Work out the finished part from the listing and answer in its coordinate system (mm). Face numbers are marked on the shaded views. A direction names the side the tool comes from. Coordinates: 2 decimals unless noted, no trailing zeros. Loops run counter-clockwise (first coordinate to the right, second up) from the corner with the lowest first, then second, coordinate; pieces in that order, holes last. Notation, with made-up numbers: (2.5, 23.25) -> (7.5, 23.25) arc R27 cw to (7.5, 54.25) -> close; hole circle Ø5 at (-2, 18). An arc over 180 degrees is marked (long way). Use a Markdown table: item, result. Add a question column.
Autodesk Inventor part; units mm, degrees
ref_plane "Work Plane1" through (-60, 0, 0) normal (1, 0, 0) x (0, 1, 0)
ref_plane "XZ Plane" through (0, 0, 0) normal (0, 1, 0) x (-1, 0, 0)
ref_plane "XY Plane" through (0, 0, 0) normal (0, 0, 1) x (1, 0, 0)
sketch "Sketch1" plane through (0, 0, 0) normal (0, 0, 1) x (1, 0, 0)
  circle A0 centre (0, 0) radius 25
  line L0 (0, 25) -> (-60, 25)
  line L1 (0, -25) -> (-60, -25)
  arc A1 (-60, 25) -> (-60, -25) centre (-60, 0) ccw
  dimension "d0" = 50
  dimension "d1" = 60
  dimension "d2" = 60
  dimension "d3" = 25
extrude "Extrusion1" add sketch "Sketch1" along normal mid plane 93
sketch "Sketch2" plane through (0, 0, 0) normal (0, 0, 1) x (1, 0, 0)
  arc A0 (0, -25) -> (0, 25) centre (0, 0) ccw
  arc A1 (-12.2474, 25) -> (-11.5542, 22.1698) centre (-12.2474, 23.5) ccw construction
  arc A2 (-11.5542, -22.1698) -> (-12.2474, -25) centre (-12.2474, -23.5) ccw construction
  line L0 (0, -25) -> (-60, -25)
  line L1 (-60, 25) -> (0, 25)
  line L2 (-12.2474, 25) -> (0, 25)
  arc A3 (0, -25) -> (0, 25) centre (0, 0) ccw
  line L3 (-12.2474, -25) -> (0, -25)
  arc A4 (-11.5542, -22.1698) -> (0, -25) centre (0, 0) ccw construction
  arc A5 (-12.2474, -25) -> (-11.5542, -22.1698) centre (-12.2474, -23.5) ccw
  arc A6 (-11.5542, 22.1698) -> (-12.2474, 25) centre (-12.2474, 23.5) ccw
  arc A7 (-11.5542, 22.1698) -> (-11.5542, -22.1698) centre (0, 0) ccw
  arc A8 (0, 25) -> (-11.5542, 22.1698) centre (0, 0) ccw construction
  dimension "d7" = 3
  dimension "d8" = 3
extrude "Extrusion2" cut sketch "Sketch2" along normal mid plane 78
sketch "Sketch3" plane through (0, 0, 0) normal (0, 0, 1) x (1, 0, 0)
  circle A0 centre (0, 0) radius 10
  dimension "d11" = 20
extrude "Extrusion3" cut sketch "Sketch3" along normal mid plane 88
sketch "Sketch4" plane through (-60, 25, -46.5) normal (0, 1, 0) x (1, 0, 0)
  line L0 (35, -7.5) -> (35, -85.5)
  line L1 (0, -93) -> (60, -93)
  line L2 (30, -93) -> (30, 0)
  line L3 (60, 0) -> (0, 0)
  line L4 (30, -93) -> (-25, -71.5)
  line L5 (-25, 0) -> (-25, -93)
  line L6 (-25, -71.5) -> (-25, -93)
  line L7 (30, -93) -> (-25, -93)
  line L8 (30, 0) -> (-25, -21.5)
  line L9 (-25, 0) -> (30, 0)
  line L10 (-25, -21.5) -> (-25, 0)
  point P0 (60, -46.5)
  dimension "d14" = 5
  dimension "d15" = 50
  dimension "d16" = 21.5
extrude "Extrusion4" cut sketch "Sketch4" against normal through all contours L7 L5 L4 L1 | L8 L5 L9 L3
ref_plane "Work Plane1" through (-60, 0, 0) normal (1, 0, 0) x (0, 1, 0)
sketch "Sketch5" plane through (-60, 0, 0) normal (1, 0, 0) x (0, 1, 0)
  circle A0 centre (0, -10) radius 25
  line L0 (-25, -46.5) -> (25, -46.5)
  line L1 (0, -46.5) -> (0, -10)
  dimension "d20" = 50
  dimension "d23" = 36.5
extrude "Extrusion5" add sketch "Sketch5" against normal blind 50
properties part number "Arm 5 v0.1"
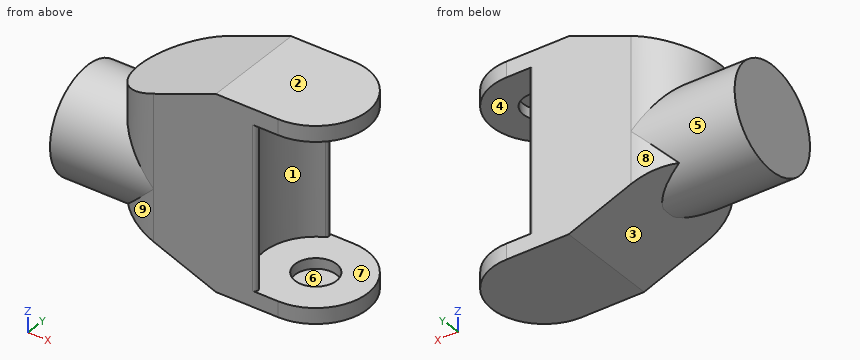
Item 1: Find the intervals of material crossed by probe 1 along Z at (x, y) = (1, 17); probe 2 along Y at (x, z) = (0, 41); probe 3 along Z at (x, y) = (-1, -5), in increasing order.
Item 2: Section B-B (y = 0) is taken. Determine the outline of the cut face in (x, z), then the cut area to 3 significant figures.
Item 3: Section D-D (z = 11) is taken. Determine the outline of the cut face in (x, y), then the cut area to 3 significant figures.
Item 4: Section A-A (x = 12) is taken. Determine the outline of the cut face in (y, z), then the cut area to 3 significant figures.
Item 5: Given pin 1 (12 mm diameter, centred on y = 6.5, z = 11, fed in from +X); pin 2 (6 mm diameter, centred on x = -60, y = 15, fed in from +Z); pin 3 (8 mm diameter, centred on x = -87, y = -3, fed in from +Z), each flat-ended and moving along its own axis, determine where each tip first touches the part or whether it passes through.
Item 6: For the marked faces 5, 6, 7, 8 and 9, determine the directions among +Z, -Z, +X, -X, +Y, -Y from which every point of the face is accessible in a straight line to the end or side of a thin tool.
Item 7: Section C-C (x = -18.5) is taken. Determine the outline of the cut face in (y, z).
Item 8: For a pull along Z with two mould halves and no side action, classify the marked faces 1, 2, 3 and 4 as +Z half, -Z half, draft (parallel to the pull), parting line (faces both ways), or undercut.
Output:
| question | item | result |
|---|---|---|
| 1 | probe 1 | z = -46.5 to -39, 39 to 46.5 |
| 1 | probe 2 | y = -25 to -10, 10 to 25 |
| 1 | probe 3 | z = -46.5 to -44, 44 to 46.5 |
| 2 | outline | (-110, -35) -> (-60, -35) -> (-60, -34.77) -> (-30, -46.5) -> (25, -46.5) -> (25, -39) -> (10, -39) -> (10, -44) -> (-10, -44) -> (-10, -39) -> (-25, -39) -> (-25, 39) -> (-10, 39) -> (-10, 44) -> (10, 44) -> (10, 39) -> (25, 39) -> (25, 46.5) -> (-30, 46.5) -> (-85, 25) -> (-85, 15) -> (-110, 15) -> close |
| 2 | area | 6,330 mm2 |
| 3 | outline | (-110, -13.56) -> (-81, -13.56) arc R25 ccw to (-60, -25) -> (-12.25, -25) arc R1.5 ccw to (-11.55, -22.17) arc R25 cw to (-11.55, 22.17) arc R1.5 ccw to (-12.25, 25) -> (-60, 25) arc R25 ccw to (-81, 13.56) -> (-110, 13.56) -> close |
| 3 | area | 3,690 mm2 |
| 4 | outline | (-21.93, -46.5) -> (21.93, -46.5) -> (21.93, -39) -> (-21.93, -39) -> close; (-21.93, 39) -> (21.93, 39) -> (21.93, 46.5) -> (-21.93, 46.5) -> close |
| 4 | area | 658 mm2 |
| 5 | pin 1 | stops at x = -21.65 |
| 5 | pin 2 | stops at z = 35.95 |
| 5 | pin 3 | stops at z = 25.78 |
| 6 | face 5 | -X |
| 6 | face 6 | none |
| 6 | face 7 | +X |
| 6 | face 8 | -Z, -X, +Y |
| 6 | face 9 | -Z, -X, -Y |
| 7 | outline | (-25, -46.5) -> (25, -46.5) -> (25, 46.5) -> (-25, 46.5) -> close; hole (-16.82, -39) -> (16.82, -39) -> (16.82, 39) -> (-16.82, 39) -> close |
| 8 | face 1 | undercut |
| 8 | face 2 | +Z half |
| 8 | face 3 | -Z half |
| 8 | face 4 | undercut |
